Answer from the drawing. Dimensions are ordinates in mm from the lowest x, y and z of the part. A direction names the side the tool comes from. Coordinates: 2 decimals unless noted, no trailing zeros. Write each loop counter-clockwise with the first axis right and the second up, starting at its lowest first coordinate (ties: lowest second). Pieces come first, ordered by that corner, then holes.
(1) The part is cut by section C-C on z = 11.5. Determine the outline of the cut face in (x, y), plus the area to 3 significant figures.
(2) Which of the six approach directions +Z, -Z, +X, -X, +Y, -Y give full straight-line access (tool end or side, diameter ignored) to the marked faces 5, 6 and 7?
(3) Straight lines are drawn through the part: line 1 (X direction, y = 10, z = 1); line 2 (Y direction, x = 12, z = 10); line 3 (X direction, y = 4, z = 18.75). For each, find the intervals that lie inside material, in ascending order.
(4) For a pull along X with two mould halves and no side action, classify the marked faces 1, 2, 3 and 4 as +X half, -X half, draft (parallel to the pull), parting line (faces both ways), or undercut.
(5) The part is cut by section B-B on x = 10. Determine the outline of the cut face in (y, z), plus the area to 3 significant figures.
(6) The part is cut by section A-A on y = 10. Determine the outline of the cut face in (x, z).
(7) The part is cut by section D-D on x = 5.5. Determine the outline of the cut face in (y, z).
(8) Given P1, Ø4, axis at y = 10, z = 10, coming from the -X side; P2, Ø1, axis at y = 2, z = 8.5, coming from the -X side; P3, Ø5, axis at y = 3, z = 5, coming from the +X side, each flat-ended and moving along its own axis, determine where each tip first touches the part or whether it passes through.
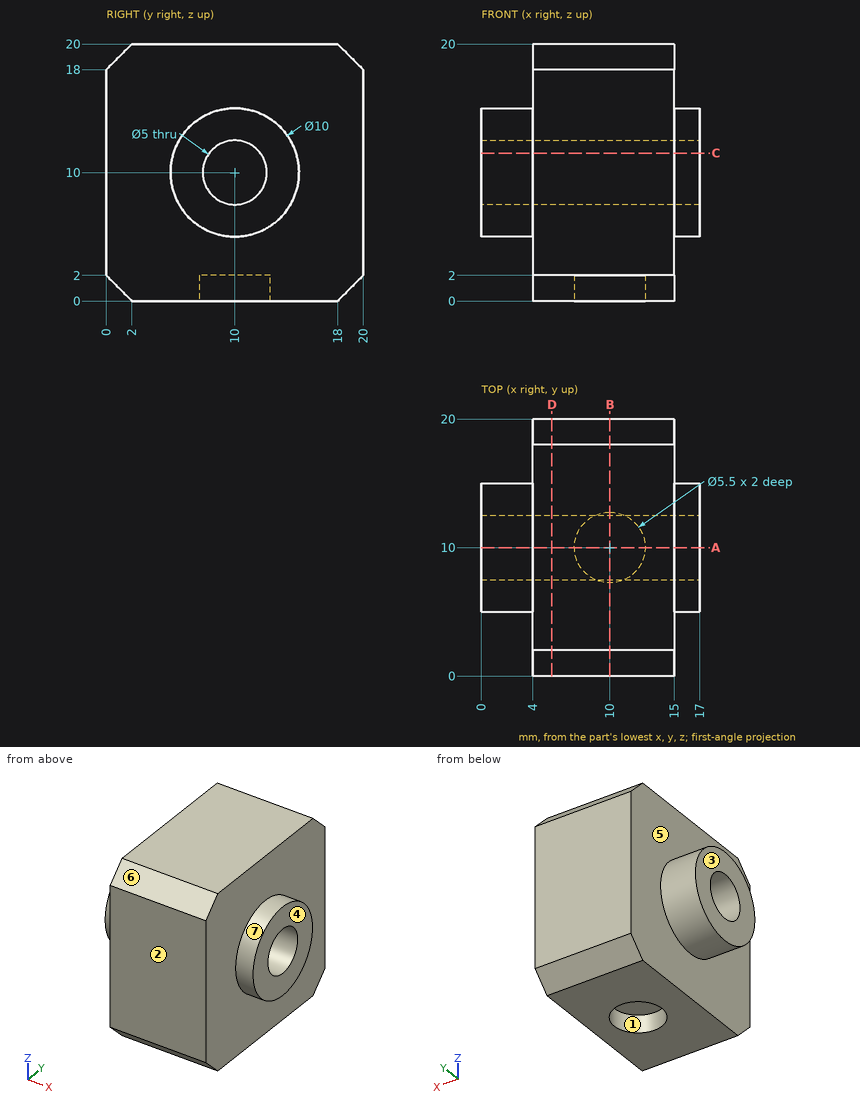
Model answer:
1. outline: (0, 5.23) - (4, 5.23) - (4, 0) - (15, 0) - (15, 5.23) - (17, 5.23) - (17, 8) - (0, 8) - close; (0, 12) - (17, 12) - (17, 14.77) - (15, 14.77) - (15, 20) - (4, 20) - (4, 14.77) - (0, 14.77) - close
1. area: 209 mm2
2. face 5: -X
2. face 6: +Z, +X, -X, -Y
2. face 7: +X
3. line 1: x = 4 to 7.25, 12.75 to 15
3. line 2: y = 0 to 7.5, 12.5 to 20
3. line 3: x = 4 to 15
4. face 1: undercut
4. face 2: draft
4. face 3: -X half
4. face 4: +X half
5. outline: (0, 2) - (2, 0) - (7.25, 0) - (7.25, 2) - (12.75, 2) - (12.75, 0) - (18, 0) - (20, 2) - (20, 18) - (18, 20) - (2, 20) - (0, 18) - close; hole circle Ø5 at (10, 10)
5. area: 361 mm2
6. outline: (0, 5) - (4, 5) - (4, 0) - (7.25, 0) - (7.25, 2) - (12.75, 2) - (12.75, 0) - (15, 0) - (15, 5) - (17, 5) - (17, 7.5) - (0, 7.5) - close; (0, 12.5) - (17, 12.5) - (17, 15) - (15, 15) - (15, 20) - (4, 20) - (4, 15) - (0, 15) - close
7. outline: (0, 2) - (2, 0) - (18, 0) - (20, 2) - (20, 18) - (18, 20) - (2, 20) - (0, 18) - close; hole circle Ø5 at (10, 10)
8. P1: passes through
8. P2: stops at x = 4
8. P3: stops at x = 15
